For this review, take the finished solid that the model builds, in its own axes (mm). A direction names the side the tool comes from. Give positions to 0.01 mm unless a question says otherwise; leave off trailing zeros. Write each loop counter-clockwise with the first axis right and the second up, starting at its lowest first coordinate (ties: lowest second). Pieces come first, ordered by that corner, then holes. Notation, with made-up numbers: M 69.5,-19 L 117.5,-19 A28 ccw 117.5,19 Z; hole C -25.5,-14 d2. An arc over 180 degrees is marked long. One line per item, written item: value. Start each with the question number.
Item 1: Mouldability with a two-part tool opening along Y and no side actions: class faces 1 (the face through (-17, 15, -1)), 2 (the face through (6, -7.5, 0)), 3 (the face through (5.4, 0.2, -20)) as released by +Y, released by -Y, zero draft, split by the parting line, or undercut.
Item 2: Clearance check with flat-ended pins moving along their axes: pin 1 Ø4 at (x, z) = (19, 6.5) entering from -Y; pin 2 Ø12 at (x, y) = (6.5, 0.5) entering from +Z; pin 3 Ø8 at (x, y) = (-6.5, -5) entering from -Z. State where each tip first meets the part, or that it passes through.
Item 3: Consider section D-D, the plane z = -5.5. Write out the cut boundary in (x, y).
Item 4: Consider section C-C, the plane z = 15. Write out the cut boundary in (x, y).
Item 5: Tool access review of faces 4 (the face through (0, -15, 0)), 5 (the face through (5.4, 0.2, 20)), 6 (the face through (-7.5, -0.16, -0.17)), 7 (the face through (-25, 17, 1)), 8 (the face through (12.5, 9, 0)): name each direction out of +Z, -Z, +X, -X, +Y, -Y from which nothing blocks a thin tool from reaching the whole face with its end or side.
Item 6: Consider section B-B, the plane x = -17. Write out the cut boundary in (y, z) (3 decimals).
Item 7: To check wall thickness, follow probe 1 along X at (y, z) = (17.35, 29.5); probe 2 along Z at (x, y) = (17, 17); probe 3 along Y at (x, z) = (0, -15). State the ranges of each line that lie inside material, in increasing order.
Item 8: Consider section A-A, the plane z = -29.5. Write out the cut boundary in (x, y) (3 decimals).
```python
from build123d import *

# Parameters (mm, degrees)
SKETCH1_W                      = 25
SKETCH1_H                      = 30
BOSS_EXTRUDE1_DEPTH            = 20
CUT_EXTRUDE1_DEPTH             = 12
CUT_EXTRUDE1_DEPTH_BACK        = 12
SKETCH3_R                      = 5
CUT_EXTRUDE2_DEPTH             = 45.511234537
SKETCH4_W                      = 50
SKETCH4_H                      = 75
BOSS_EXTRUDE2_DEPTH            = 5
FILLET1_R                      = 10
M4_CLEARANCE_HOLE1_D           = 4.5
M4_CLEARANCE_HOLE1_CSINK_D     = 4.55
M4_CLEARANCE_HOLE1_CSINK_ANGLE = 90


with BuildPart() as part:
    # Sketch1 → Boss-Extrude1 (new, symmetric)
    with BuildSketch(Plane.XY):
        Rectangle(SKETCH1_W, SKETCH1_H)
    extrude(amount=BOSS_EXTRUDE1_DEPTH, both=True)

    # Sketch2 → Cut-Extrude1 (cut, two sides: drawn at the far end of the back side and taken through both)
    with BuildSketch(Plane.XY.offset(-CUT_EXTRUDE1_DEPTH_BACK)):
        with BuildLine():
            Line((0, 7.5), (21.39891064, 7.5))
            Line((21.39891064, 7.5), (21.39891064, -7.5))
            Line((21.39891064, -7.5), (0, -7.5))
            ThreePointArc((0, -7.5), (-7.5, 0), (0, 7.5))
        make_face()
    extrude(amount=CUT_EXTRUDE1_DEPTH + CUT_EXTRUDE1_DEPTH_BACK, mode=Mode.SUBTRACT)

    # Sketch3 → Cut-Extrude2 (cut, through all)
    with BuildSketch(Plane.XY.offset(20)):
        Circle(SKETCH3_R)
    extrude(amount=-CUT_EXTRUDE2_DEPTH, mode=Mode.SUBTRACT)

    # Sketch4 → Boss-Extrude2 (add)
    with BuildSketch(Plane(origin=(0, 15, 0), x_dir=(1, 0, 0), z_dir=(0, 1, 0))):
        Rectangle(SKETCH4_W, SKETCH4_H)
    extrude(amount=BOSS_EXTRUDE2_DEPTH)

    # Fillet1
    # the kernel refuses this fillet: 10 mm, written as the material it takes off along each edge
    with BuildSketch(Plane(origin=(-12.5, -15, 45), x_dir=(0, 1, 0), z_dir=(0, 0, -1)), Plane(origin=(12.5, -15, -45), x_dir=(0, 1, 0), z_dir=(0, 0, 1))) as fillet1_piece_1:
        with BuildLine():
            CenterArc((FILLET1_R, FILLET1_R), FILLET1_R, 180, 90)
            Line((0, FILLET1_R), (0, 0))
            Line((0, 0), (FILLET1_R, 0))
        make_face()
    extrude(amount=90, mode=Mode.SUBTRACT)

    # M4 Clearance Hole1 (through all)
    with Locations(Plane(origin=(0, 15, 0), x_dir=(-1, 0, 0), z_dir=(0, -1, 0))):
        with Locations((-17, 29.5), (17, 29.5), (17, -29.5), (-17, -29.5)):
            CounterSinkHole(M4_CLEARANCE_HOLE1_D / 2, M4_CLEARANCE_HOLE1_CSINK_D / 2, counter_sink_angle=M4_CLEARANCE_HOLE1_CSINK_ANGLE)


solid = part.part
```
Model answer:
1. face 1: released by -Y
1. face 2: undercut
1. face 3: zero draft
2. pin 1: stops at y = 15
2. pin 2: stops at z = 20
2. pin 3: stops at z = -20
3. outline: M -25,15 L -12.5,15 L -12.5,-5 A10 ccw -2.5,-15 L 2.5,-15 A10 ccw 12.18,-7.5 L 0,-7.5 A7.5 cw 0,7.5 L 12.5,7.5 L 12.5,15 L 25,15 L 25,20 L -25,20 Z
4. outline: M -25,15 L -12.5,15 L -12.5,-5 A10 ccw -2.5,-15 L 2.5,-15 A10 ccw 12.5,-5 L 12.5,15 L 25,15 L 25,20 L -25,20 Z; hole C 0,0 d10
5. face 4: +Z, -Z, +X, -X, -Y
5. face 5: +Z, +X, -X, -Y
5. face 6: +X
5. face 7: +Z, -Z, -X, +Y, -Y
5. face 8: +Z, -Z, +X, -Y
6. outline: M 15,-37.5 L 20,-37.5 L 20,-31.75 L 15.025,-31.75 L 15,-31.775 Z; M 15,-27.225 L 15.025,-27.25 L 20,-27.25 L 20,27.25 L 15.025,27.25 L 15,27.225 Z; M 15,31.775 L 15.025,31.75 L 20,31.75 L 20,37.5 L 15,37.5 Z
7. probe 1: x = -25 to -19.25, -14.75 to 14.75, 19.25 to 25
7. probe 2: z = -37.5 to -31.75, -27.25 to 27.25, 31.75 to 37.5
7. probe 3: y = -15 to -5, 5 to 20
8. outline: M -25,15 L -19.275,15 L -19.25,15.025 L -19.25,20 L -25,20 Z; M -14.75,15.025 L -14.725,15 L 14.725,15 L 14.75,15.025 L 14.75,20 L -14.75,20 Z; M 19.25,15.025 L 19.275,15 L 25,15 L 25,20 L 19.25,20 Z
